Could you check a few things on this model? Use its own coordinates, in mm. Round coordinates to 2 decimals unless told otherwise and drop trailing zeros. Loops run counter-clockwise (first coordinate to the right, second up) from the corner with the lowest first, then second, coordinate; pieces in that order, holes last. Notation, with made-up numbers: M 79.25,80.25 L 129.25,80.25 A28 ccw 129.25,108.25 Z; hole C -13,71.25 d4. An arc over 180 degrees is marked long. Answer in a Markdown table with one row per item.
```python
from build123d import *

# Parameters (mm, degrees)
SKETCH1_W           = 530
SKETCH1_H           = 635
BOSS_EXTRUDE1_DEPTH = 3
SKETCH2_R           = 1.5
CUT_EXTRUDE1_DEPTH  = 586.517705704
SKETCH3_R           = 2.5
SKETCH3_R_2         = 1.5
CUT_EXTRUDE2_DEPTH  = 586.517705704
SKETCH13_W          = 141
SKETCH13_H          = 141
CUT_EXTRUDE20_DEPTH = 2
SKETCH14_R          = 2.085
SKETCH14_R_2        = 68
CUT_EXTRUDE21_DEPTH = 586.513435963
SKETCH15_R          = 2.085
SKETCH15_R_2        = 68
CUT_EXTRUDE22_DEPTH = 586.513435963


with BuildPart() as part:
    # Sketch1 → Boss-Extrude1 (new body)
    with BuildSketch(Plane.XY):
        with Locations((-211.504854369, -22.742718447)):
            Rectangle(SKETCH1_W, SKETCH1_H)
    extrude(amount=BOSS_EXTRUDE1_DEPTH)

    # Sketch2 → Cut-Extrude1 (cut, through all)
    with BuildSketch(Plane.XY.offset(3)):
        with Locations((-452.244854369, 231.757281553)):
            Circle(SKETCH2_R)
        with Locations((-452.244854369, 223.757281553)):
            Circle(SKETCH2_R)
        with Locations((-452.244854369, 215.757281553)):
            Circle(SKETCH2_R)
        with Locations((-452.244854369, -278.242718447)):
            Circle(SKETCH2_R)
        with Locations((-452.244854369, -286.242718447)):
            Circle(SKETCH2_R)
        with Locations((-452.244854369, -294.242718447)):
            Circle(SKETCH2_R)
    extrude(amount=-CUT_EXTRUDE1_DEPTH, mode=Mode.SUBTRACT)

    # Sketch3 → Cut-Extrude2 (cut, through all)
    with BuildSketch(Plane.XY.offset(3)):
        with Locations((8.495145631, 69.757281553)):
            Circle(SKETCH3_R)
        with Locations((8.495145631, 53.757281553)):
            Circle(SKETCH3_R)
        with Locations((8.495145631, -99.242718447)):
            Circle(SKETCH3_R)
        with Locations((8.495145631, -115.242718447)):
            Circle(SKETCH3_R)
        with Locations((8.495145631, -8.242718447)):
            Circle(SKETCH3_R_2)
        with Locations((8.495145631, -37.242718447)):
            Circle(SKETCH3_R_2)
    extrude(amount=-CUT_EXTRUDE2_DEPTH, mode=Mode.SUBTRACT)

    # Sketch13 → Cut-Extrude20 (cut)
    with BuildSketch(Plane(origin=(0, 0, 0), x_dir=(-1, 0, 0), z_dir=(0, 0, -1))):
        with Locations((105.504854369, -22.742718447)):
            Rectangle(SKETCH13_W, SKETCH13_H)
        with Locations((317.504854369, -22.742718447)):
            Rectangle(SKETCH13_W, SKETCH13_H)
    extrude(amount=-CUT_EXTRUDE20_DEPTH, mode=Mode.SUBTRACT)

    # Sketch14 → Cut-Extrude21 (cut, through all)
    with BuildSketch(Plane(origin=(0, 0, 2), x_dir=(-1, 0, 0), z_dir=(0, 0, -1))):
        with Locations((43.004854369, 39.757281553)):
            Circle(SKETCH14_R)
        with Locations((168.004854369, 39.757281553)):
            Circle(SKETCH14_R)
        with Locations((43.004854369, -85.242718447)):
            Circle(SKETCH14_R)
        with Locations((168.004854369, -85.242718447)):
            Circle(SKETCH14_R)
        with Locations((105.504854369, -22.742718447)):
            Circle(SKETCH14_R_2)
    extrude(amount=-CUT_EXTRUDE21_DEPTH, mode=Mode.SUBTRACT)

    # Sketch15 → Cut-Extrude22 (cut, through all)
    with BuildSketch(Plane(origin=(0, 0, 2), x_dir=(-1, 0, 0), z_dir=(0, 0, -1))):
        with Locations((255.004854369, 39.757281553)):
            Circle(SKETCH15_R)
        with Locations((380.004854369, 39.757281553)):
            Circle(SKETCH15_R)
        with Locations((255.004854369, -85.242718447)):
            Circle(SKETCH15_R)
        with Locations((380.004854369, -85.242718447)):
            Circle(SKETCH15_R)
        with Locations((317.504854369, -22.80647888)):
            Circle(SKETCH15_R_2)
    extrude(amount=-CUT_EXTRUDE22_DEPTH, mode=Mode.SUBTRACT)


solid = part.part
```
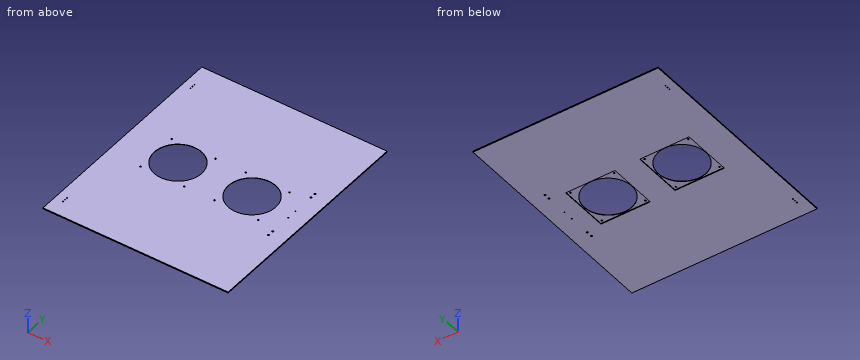
1) I want a section at A-A, the plane x = -288. Please give me the cut outline in (y, z).
Computed:
| item | result |
|---|---|
| outline | M -340.24,0 L -93.24,0 L -93.24,2 L -84.07,2 L -84.07,3 L -340.24,3 Z; M 38.46,2 L 47.76,2 L 47.76,0 L 294.76,0 L 294.76,3 L 38.46,3 Z |
2) I want a section at C-C, the plane y = 2.5. Please give me the cut outline in (x, z).
Computed:
| item | result |
|---|---|
| outline | M -476.5,0 L -388,0 L -388,2 L -380.62,2 L -380.62,3 L -476.5,3 Z; M -254.39,2 L -247,2 L -247,0 L -176,0 L -176,2 L -168.65,2 L -168.65,3 L -254.39,3 Z; M -42.36,2 L -35,2 L -35,0 L 53.5,0 L 53.5,3 L -42.36,3 Z |
3) I need wall thicknesses on line 1 (X direction, y = -65.5, z = 1.5); line 2 (Y direction, x = -95.5, z = 1.4); line 3 (Y direction, x = -43.5, z = 2.5). Which ranges of each line are inside material? Lowest first, please.
Computed:
| item | result |
|---|---|
| line 1 | x = -476.5 to -388, -247 to -176, -35 to 53.5 |
| line 2 | y = -340.24 to -93.24, 47.76 to 294.76 |
| line 3 | y = -340.24 to -87.27, -83.22 to -50.66, 5.17 to 37.73, 41.78 to 294.76 |
4) Will these pins go through, and if not, where does the flat tip stop? P1, Ø4, axis at x = 8.5, y = 53.76, coming from the -Z side; P2, Ø5, axis at x = -380, y = 39.76, coming from the -Z side.
Computed:
| item | result |
|---|---|
| P1 | passes through |
| P2 | stops at z = 2 |
5) I want a section at B-B, the plane z = 1.3. State how many separate pieces and enclosed holes the cut face has, plus the area to 3 significant figures.
Computed:
| item | result |
|---|---|
| separate pieces | 1 |
| enclosed holes | 14 |
| area | 297,000 mm² |
